```python
from build123d import *

# Parameters (mm, degrees)
SKETCH1_W                       = 279.4
SKETCH1_H                       = 76.2
BOSS_EXTRUDE1_DEPTH             = 3
SKETCH3_W                       = 3
SKETCH3_H                       = 15
CUT_EXTRUDE1_DEPTH              = 145.833352512
LPATTERN1_COUNT                 = 3
LPATTERN1_PITCH                 = 22.8
MIRROR1_COPY_1_SKETCH_W         = 3
MIRROR1_COPY_1_SKETCH_H         = 15
MIRROR1_COPY_1_DEPTH            = 145.833352512
MIRROR1_COPY_2_SKETCH_W         = 3
MIRROR1_COPY_2_SKETCH_H         = 15
MIRROR1_COPY_2_DEPTH            = 145.833352512
F_3_0MM_CLEARANCE_DOWEL_HOLE1_D = 3


with BuildPart() as part:
    # Sketch1 → Boss-Extrude1 (new body)
    with BuildSketch(Plane(origin=(0, 0, 0), x_dir=(0, 0, -1), z_dir=(1, 0, 0))):
        Rectangle(SKETCH1_W, SKETCH1_H)
    extrude(amount=-BOSS_EXTRUDE1_DEPTH)

    # Sketch3 → Cut-Extrude1 (cut, through all)
    with BuildSketch(Plane.ZY.offset(3)):
        with Locations((133.2, 22.8)):
            Rectangle(SKETCH3_W, SKETCH3_H)
    cut_extrude1 = extrude(amount=-CUT_EXTRUDE1_DEPTH, mode=Mode.SUBTRACT)

    # LPattern1: Cut-Extrude1 ×3
    with Locations(*[(0, -i * LPATTERN1_PITCH, 0) for i in range(1, LPATTERN1_COUNT)]):
        add(cut_extrude1, mode=Mode.SUBTRACT)

    # Mirror1: Cut-Extrude1 across plane
    add(cut_extrude1.mirror(Plane.XY), mode=Mode.SUBTRACT)

    # Mirror1 copy 1 sketch → Mirror1 copy 1 (cut, through all)
    with BuildSketch(Plane(origin=(-3, -22.8, 0), x_dir=(0, 0, -1), z_dir=(-1, 0, 0))):
        with Locations((133.2, -22.8)):
            Rectangle(MIRROR1_COPY_1_SKETCH_W, MIRROR1_COPY_1_SKETCH_H)
    extrude(amount=-MIRROR1_COPY_1_DEPTH, mode=Mode.SUBTRACT)

    # Mirror1 copy 2 sketch → Mirror1 copy 2 (cut, through all)
    with BuildSketch(Plane(origin=(-3, -45.6, 0), x_dir=(0, 0, -1), z_dir=(-1, 0, 0))):
        with Locations((133.2, -22.8)):
            Rectangle(MIRROR1_COPY_2_SKETCH_W, MIRROR1_COPY_2_SKETCH_H)
    extrude(amount=-MIRROR1_COPY_2_DEPTH, mode=Mode.SUBTRACT)

    # Ø3.0mm Clearance Dowel Hole1 (through all)
    with Locations(Plane.ZY.offset(3)):
        with Locations((-69.85, 0), (69.85, 0)):
            Hole(F_3_0MM_CLEARANCE_DOWEL_HOLE1_D / 2)


solid = part.part
```
For this review, take the finished solid that the model builds, in its own axes (mm). Round coordinates to 2 decimals unless told otherwise and drop trailing zeros. Order: outer loops, then holes, each group sorted by start corner. A loop starts at its lowest first (then second) coordinate and runs counter-clockwise, first axis right, second up.
Q1. Wall thickness on line 1 (Z direction, x = -0.2, y = -22); line 2 (Y direction, x = -1.7, z = 69.85): over which ranges is each line inside the solid? List them lowest first.
Findings below:
line 1: z = -139.7 to -134.7, -131.7 to 131.7, 134.7 to 139.7
line 2: y = -38.1 to -1.5, 1.5 to 38.1
Q2. Insertion check: P1, Ø2.5, axis at y = 0, z = 69.85, coming from the +X side. The pin has a flat end and moves straight along its axis. Give the tip position at first contact, or say it passes through.
Findings below:
P1: passes through
Q3. We need section A-A, the plane y = -21. Give the boundary of the cut face in (x, z), plus the area to 3 significant figures.
Findings below:
outline: (-3, -139.7) - (0, -139.7) - (0, -134.7) - (-3, -134.7) - close; (-3, -131.7) - (0, -131.7) - (0, 131.7) - (-3, 131.7) - close; (-3, 134.7) - (0, 134.7) - (0, 139.7) - (-3, 139.7) - close
area: 820 mm2
Q4. Mouldability with a two-part tool opening along X and no side actions: class faces 1 (the flat face through (-3, 1, 2)), 2 (the flat face through (0, 1, 2)) as pulls with the +X half, pulls with the -X half, needs draft (parallel to the pull), parting line crosses it, or undercut.
Findings below:
face 1: pulls with the -X half
face 2: pulls with the +X half
